Work out the finished part from the listing and answer in its coordinate system (mm). Face numbers are marked on the shaded views. A direction names the side the tool comes from. Round coordinates to 2 decimals unless told otherwise and drop trailing zeros. Loops run counter-clockwise (first coordinate to the right, second up) from the corner with the lowest first, then second, coordinate; pieces in that order, holes last.
from build123d import *

# Parameters (mm, degrees)
BOSS_EXTRUDE1_DEPTH = 25.4
SKETCH2_W           = 44.704
SKETCH2_H           = 0.0254
CUT_EXTRUDE1_DEPTH  = 107.377492525
SKETCH3_R           = 2.286
CUT_EXTRUDE2_DEPTH  = 107.377492525
CUT_EXTRUDE3_DEPTH  = 109.360401051


# Read off the part's stored shape, not the designer's step: 1/4 NPT Tapped Hole1
with BuildPart() as part:
    # Sketch1 → Boss-Extrude1 (new body)
    with BuildSketch(Plane(origin=(0, 0, 0), x_dir=(1, 0, 0), z_dir=(0, 1, 0))):
        Polygon((44.704, -5.08), (95.504, -5.08), (95.504, 39.37), (0, 39.37), (0, 0), (44.704, 0), align=None)
    extrude(amount=BOSS_EXTRUDE1_DEPTH)

    # Sketch2 → Cut-Extrude1 (cut, through all)
    with BuildSketch(Plane.XY):
        with Locations((22.352, 25.3873)):
            Rectangle(SKETCH2_W, SKETCH2_H)
        with Locations((22.352, 0.0127)):
            Rectangle(SKETCH2_W, SKETCH2_H)
    extrude(amount=-CUT_EXTRUDE1_DEPTH, mode=Mode.SUBTRACT)

    # Sketch3 → Cut-Extrude2 (cut, through all)
    with BuildSketch(Plane(origin=(0, 25.4, 0), x_dir=(1, 0, 0), z_dir=(0, 1, 0))):
        with Locations(Location((49.784, 0, 0), (0, 0, 270))):
            Circle(SKETCH3_R)
        with Locations(Location((84.328, 34.544, 0), (0, 0, 270))):
            Circle(SKETCH3_R)
    extrude(amount=-CUT_EXTRUDE2_DEPTH, mode=Mode.SUBTRACT)

    # 1/4 NPT Tapped Hole1 outline → 1/4 NPT Tapped Hole1 (revolve, cut)
    with BuildSketch(Plane(origin=(69.85, 12.7, 0), x_dir=(1, 0, 0), z_dir=(0, -1, 0))):
        Polygon((5.5626, -22.352), (0, -19.009652721), (0, -39.37), (6.8545837, -39.37), (6.557984794, -29.464), (5.5626, -29.464), align=None)
    revolve(axis=Axis((69.85, 12.7, 0), (0, 0, 1)), mode=Mode.SUBTRACT)

    # 1_4 NPT Tapped Hole1 2 outline → 1_4 NPT Tapped Hole1 2 (revolve, cut)
    with BuildSketch(Plane(origin=(82.042, 12.7, 0), x_dir=(1, 0, 0), z_dir=(0, -1, 0))):
        Polygon((0, 5.08), (0, -15.280347279), (5.5626, -11.938), (5.5626, -4.826), (6.557984794, -4.826), (6.8545837, 5.08), align=None)
    revolve(axis=Axis((82.042, 12.7, 0), (0, 0, 1)), mode=Mode.SUBTRACT)

    # 1_4 NPT Tapped Hole1 3 outline → 1_4 NPT Tapped Hole1 3 (revolve, cut)
    with BuildSketch(Plane(origin=(59.944, 12.7, 0), x_dir=(1, 0, 0), z_dir=(0, -1, 0))):
        Polygon((6.8545837, 5.08), (0, 5.08), (0, -15.280347279), (5.5626, -11.938), (5.5626, -4.826), (6.557984794, -4.826), align=None)
    revolve(axis=Axis((59.944, 12.7, 0), (0, 0, 1)), mode=Mode.SUBTRACT)

    # Sketch7 → Cut-Extrude3 (cut, through all)
    with BuildSketch(Plane.XY.offset(5.08)):
        Polygon((95.504, 25.4), (95.504, 17.78), (91.660260387, 25.4), align=None)
        Polygon((91.660260387, 0), (95.504, 0), (95.504, 7.62), align=None)
    extrude(amount=-CUT_EXTRUDE3_DEPTH, mode=Mode.SUBTRACT)


solid = part.part
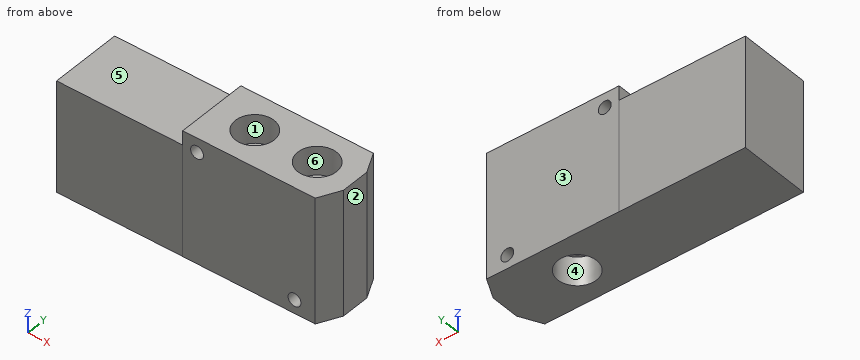
Item 1: Section A-A, the plane z = -10 is taken. State how many separate pieces and enclosed holes the cut face has, plus the area to 3 significant figures.
Item 2: For the marked faces 4, 5 and 6, determine the directions among +Z, -Z, +X, -X, +Y, -Y from which every point of the face is accessible in a straight line to the end or side of a thin tool.
Item 3: Each of these flat-tipped pins is pushed along its axis until it touches: P1, Ø12.5, axis at x = 32, y = 11.5, coming from the +Z side; P2, Ø4, axis at x = 17.5, z = -1.5, coming from the +Y side; P3, Ø13, axis at x = 82.042, y = 12.7, coming from the +Z side. Where does it stop, or does it pass through?
Item 4: Section C-C, the plane x = 20 is taken. Give the vertices of the cut face in (y, z), plus the area to 3 significant figures.
Item 5: Straight lines are drawn through the part: line 1 (X direction, y = 10, z = -3); line 2 (Y direction, x = 11.5, z = -28); line 3 (Y direction, x = 86, z = -0.5). For each, find the intervals that lie inside material, in ascending order.
Item 6: Determine the mould class of the marked faces 1, 2 and 3 for opening direction Y: pulls with the +Y half, pulls with the -Y half, needs draft (parallel to the pull), parting line crosses it, or undercut.
Answer below:
1. separate pieces: 1
1. enclosed holes: 2
1. area: 2,200 mm2
2. face 4: -Z
2. face 5: +Z, -X, +Y, -Y
2. face 6: +Z
3. P1: stops at z = 0
3. P2: stops at y = 25.37
3. P3: stops at z = -4.83
4. outline: (0.03, -39.37) - (25.37, -39.37) - (25.37, 0) - (0.03, 0) - close
4. area: 998 mm2
5. line 1: x = 0 to 53.91, 65.98 to 76.01, 88.08 to 95.5
5. line 2: y = 0.03 to 25.37
5. line 3: y = 0 to 7.31, 18.09 to 25.4
6. face 1: undercut
6. face 2: needs draft
6. face 3: pulls with the +Y half
